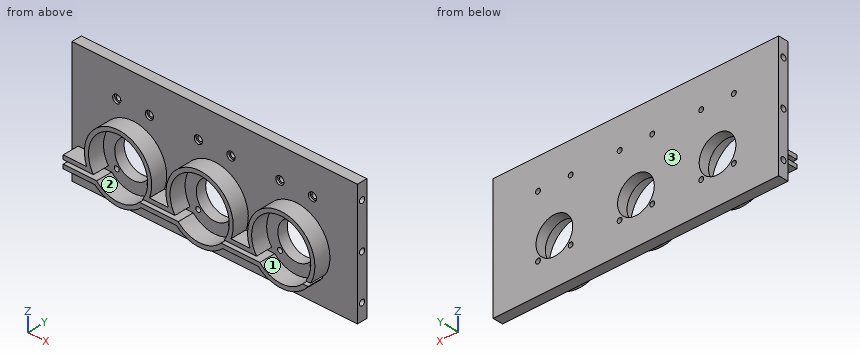
from build123d import *

# Parameters (mm, degrees)
SKETCH_1_W             = 140
SKETCH_1_H             = 60
EXTRUDE_1_DEPTH        = 5
SKETCH_2_R             = 1.2
SKETCH_2_R_2           = 9
CUT_EXTRUDE_872_DEPTH  = 153.397506541
SKETCH_4_R             = 1.4
CUT_EXTRUDE_3_DEPTH    = 5
PATTERN_LINEAR_1_COUNT = 3
PATTERN_LINEAR_1_PITCH = 40
EXTRUDE_5_DEPTH        = 8
SKETCH_6_R             = 2
CUT_EXTRUDE_4_DEPTH    = 1


with BuildPart() as part:
    # Sketch 1 → Extrude 1 (new body)
    with BuildSketch(Plane(origin=(0, 0, 0), x_dir=(1, 0, 0), z_dir=(0, 1, 0))):
        with Locations((70, -30)):
            Rectangle(SKETCH_1_W, SKETCH_1_H)
    extrude(amount=EXTRUDE_1_DEPTH)

    # Sketch 2 → Cut-Extrude 872 (cut, through all)
    with BuildSketch(Plane(origin=(0, 5, 0), x_dir=(1, 0, 0), z_dir=(0, 1, 0))):
        with Locations(Location((102, -15, 0), (0, 0, 270))):
            Circle(SKETCH_2_R)
        with Locations(Location((118, -15, 0), (0, 0, 270))):
            Circle(SKETCH_2_R)
        with Locations(Location((102, -45, 0), (0, 0, 90))):
            Circle(SKETCH_2_R)
        with Locations(Location((118, -45, 0), (0, 0, 90))):
            Circle(SKETCH_2_R)
        with Locations(Location((110, -22.5, 0), (0, 0, 270))):
            Circle(SKETCH_2_R_2)
    cut_extrude_872 = extrude(amount=-CUT_EXTRUDE_872_DEPTH, mode=Mode.SUBTRACT)

    # Sketch 4 → Cut-Extrude 3 (cut)
    with BuildSketch(Plane.ZY):
        with Locations((30, 2.5)):
            Circle(SKETCH_4_R)
        with Locations((8, 2.5)):
            Circle(SKETCH_4_R)
        with Locations((52, 2.5)):
            Circle(SKETCH_4_R)
    cut_extrude_3 = extrude(amount=-CUT_EXTRUDE_3_DEPTH, mode=Mode.SUBTRACT)

    # Mirror 1: Cut-Extrude 3 across plane
    add(cut_extrude_3.mirror(Plane(origin=(70, 0, 0), x_dir=(0, 0, 1), z_dir=(1, 0, 0))), mode=Mode.SUBTRACT)

    # Pattern Linear 1: Cut-Extrude 872 ×3
    with Locations(*[(-i * PATTERN_LINEAR_1_PITCH, 0, 0) for i in range(1, PATTERN_LINEAR_1_COUNT)]):
        add(cut_extrude_872, mode=Mode.SUBTRACT)

    # Sketch 5 → Extrude 5 (add)
    with BuildSketch(Plane.XZ):
        with BuildLine():
            Line((15.56913031, 14.5), (17.906613378, 14.5))
            ThreePointArc((17.906613378, 14.5), (30, 37), (42.093386622, 14.5))
            Line((42.093386622, 14.5), (55.56913031, 14.5))
            Line((55.56913031, 14.5), (57.906613378, 14.5))
            ThreePointArc((57.906613378, 14.5), (70, 37), (82.093386622, 14.5))
            Line((82.093386622, 14.5), (95.56913031, 14.5))
            Line((95.56913031, 14.5), (97.906613378, 14.5))
            ThreePointArc((97.906613378, 14.5), (110, 37), (122.093386622, 14.5))
            Line((122.093386622, 14.5), (124.43086969, 14.5))
            ThreePointArc((124.43086969, 14.5), (111.104849123, 38.962967789), (94.629573851, 16.5))
            Line((94.629573851, 16.5), (85.370426149, 16.5))
            ThreePointArc((85.370426149, 16.5), (70, 39), (54.629573851, 16.5))
            Line((54.629573851, 16.5), (45.370426149, 16.5))
            ThreePointArc((45.370426149, 16.5), (30, 39), (14.629573851, 16.5))
            Line((14.629573851, 16.5), (3.1, 16.5))
            Line((3.1, 16.5), (3.1, 14.5))
            Line((3.1, 14.5), (15.56913031, 14.5))
        make_face()
        with BuildLine():
            Line((16.875595252, 12.5), (19.5, 12.5))
            ThreePointArc((19.5, 12.5), (30, 8), (40.5, 12.5))
            Line((40.5, 12.5), (56.875595252, 12.5))
            Line((56.875595252, 12.5), (59.5, 12.5))
            ThreePointArc((59.5, 12.5), (70, 8), (80.5, 12.5))
            Line((80.5, 12.5), (96.875595252, 12.5))
            Line((96.875595252, 12.5), (99.5, 12.5))
            ThreePointArc((99.5, 12.5), (110, 8), (120.5, 12.5))
            Line((120.5, 12.5), (123.124404748, 12.5))
            ThreePointArc((123.124404748, 12.5), (111.345246377, 6.05493046), (98.675248347, 10.5))
            Line((98.675248347, 10.5), (81.324751653, 10.5))
            ThreePointArc((81.324751653, 10.5), (70, 6), (58.675248347, 10.5))
            Line((58.675248347, 10.5), (41.324751653, 10.5))
            ThreePointArc((41.324751653, 10.5), (30, 6), (18.675248347, 10.5))
            Line((18.675248347, 10.5), (3.1, 10.5))
            Line((3.1, 10.5), (3.1, 12.5))
            Line((3.1, 12.5), (16.875595252, 12.5))
        make_face()
    extrude(amount=EXTRUDE_5_DEPTH)

    # Sketch 6 → Cut-Extrude 4 (cut)
    with BuildSketch(Plane.XZ):
        with Locations(Location((22, 45, 0), (0, 0, 270))):
            Circle(SKETCH_6_R)
        with Locations(Location((38, 45, 0), (0, 0, 270))):
            Circle(SKETCH_6_R)
        with Locations(Location((62, 45, 0), (0, 0, 270))):
            Circle(SKETCH_6_R)
        with Locations(Location((78, 45, 0), (0, 0, 270))):
            Circle(SKETCH_6_R)
        with Locations(Location((102, 45, 0), (0, 0, 270))):
            Circle(SKETCH_6_R)
        with Locations(Location((118, 45, 0), (0, 0, 270))):
            Circle(SKETCH_6_R)
    extrude(amount=-CUT_EXTRUDE_4_DEPTH, mode=Mode.SUBTRACT)


solid = part.part
Geometry: final body of the model. Coordinates: model frame, mm. Face numbers are marked on the shaded views. Coordinates: 2 decimals unless noted, no trailing zeros. Write each loop counter-clockwise with the first axis right and the second up, starting at its lowest first coordinate (ties: lowest second). Pieces come first, ordered by that corner, then holes. Notation, with made-up numbers: (-20.75, -32.75) - (-5.75, -32.75) arc R25 cw to (-5.75, -18.75) - close; hole circle Ø3 at (15.25, 50). An arc over 180 degrees is marked (long way). Return JSON: item names as keys, results as strings.
Item 1: Section query C-C (x = 9). Output: boundary loops of the cut face in (y, z), and give its area (3 significant figures).
Completed:
{"outline": "(-8, 10.5) - (0, 10.5) - (0, 0) - (5, 0) - (5, 60) - (0, 60) - (0, 16.5) - (-8, 16.5) - (-8, 14.5) - (0, 14.5) - (0, 12.5) - (-8, 12.5) - close", "area": "332 mm2"}
Item 2: Pin query (flat end, axial travel): pin 1 Ø3 at (x, y) = (37, -3) entering from +Z; pin 2 Ø6 at (x, z) = (104, 52) entering from -Y; pin 3 Ø4 at (x, y) = (45.5, -3) entering from +Z. Return the tip coordinate at first contact, or that it passes through.
Completed:
{"pin 1": "stops at z = 38.06", "pin 2": "stops at y = 0", "pin 3": "stops at z = 31.99"}
Item 3: Section query B-B (x = 110). Output: boundary loops of the cut face in (y, z), and give its area (3 significant figures).
Completed:
{"outline": "(-8, 6) - (0, 6) - (0, 0) - (5, 0) - (5, 13.5) - (0, 13.5) - (0, 8) - (-8, 8) - close; (-8, 37) - (0, 37) - (0, 31.5) - (5, 31.5) - (5, 60) - (0, 60) - (0, 39) - (-8, 39) - close", "area": "242 mm2"}
Item 4: Line query: L1, parallel to X at y = 2.2, z = 22.5; L2, parallel to Z at x = 50.5, y = -5; L3, parallel to X at y = -6, z = 37.5. Output: solid intervals per line, ascending.
Completed:
{"L1": "x = 0 to 21, 39 to 61, 79 to 101, 119 to 140", "L2": "z = 10.5 to 12.5, 14.5 to 16.5", "L3": "x = 23.13 to 36.87, 63.13 to 76.87, 103.13 to 116.87"}
Item 5: Section query A-A (y = -3). Output: boundary loops of the cut face in (x, z), and give its area (3 significant figures).
Completed:
{"outline": "(3.1, 10.5) - (18.68, 10.5) arc R16.5 ccw to (41.32, 10.5) - (58.68, 10.5) arc R16.5 ccw to (81.32, 10.5) - (98.68, 10.5) arc R16.5 ccw to (123.12, 12.5) - (120.5, 12.5) arc R14.5 cw to (99.5, 12.5) - (80.5, 12.5) arc R14.5 cw to (59.5, 12.5) - (40.5, 12.5) arc R14.5 cw to (19.5, 12.5) - (3.1, 12.5) - close; (3.1, 14.5) - (17.91, 14.5) arc R14.5 cw (long way) to (42.09, 14.5) - (57.91, 14.5) arc R14.5 cw (long way) to (82.09, 14.5) - (97.91, 14.5) arc R14.5 cw (long way) to (122.09, 14.5) - (124.43, 14.5) arc R16.5 ccw (long way) to (94.63, 16.5) - (85.37, 16.5) arc R16.5 ccw (long way) to (54.63, 16.5) - (45.37, 16.5) arc R16.5 ccw (long way) to (14.63, 16.5) - (3.1, 16.5) - close", "area": "710 mm2"}
Item 6: Section query D-D (z = 22.5). Count the separate pieces of the cut face and the enclosed holes in it, and give its area (3 significant figures).
Completed:
{"separate pieces": "4", "enclosed holes": "0", "area": "526 mm2"}
Item 7: Pull-direction query (Z, two-part tool) for the marked faces 1, 2 and 3; classes: +Z half, -Z half, draft (parallel to the pull), parting line (faces both ways), or undercut.
Completed:
{"face 1": "undercut", "face 2": "undercut", "face 3": "draft"}
